from build123d import *

# Parameters (mm, degrees)
SKETCH1_W           = 180
SKETCH1_H           = 70
BOSS_EXTRUDE1_DEPTH = 3
SKETCH2_W           = 3
SKETCH2_H           = 27
SKETCH2_W_2         = 40
SKETCH2_H_2         = 3
CUT_EXTRUDE6_DEPTH  = 10
SKETCH3_R           = 5
CUT_EXTRUDE7_DEPTH  = 12


with BuildPart() as part:
    # Sketch1 → Boss-Extrude1 (new body)
    with BuildSketch(Plane(origin=(0, 0, 0), x_dir=(0, 0, -1), z_dir=(1, 0, 0))):
        Rectangle(SKETCH1_W, SKETCH1_H)
    extrude(amount=BOSS_EXTRUDE1_DEPTH)

    # Sketch2 → Cut-Extrude6 (cut)
    with BuildSketch(Plane(origin=(3, 0, 0), x_dir=(0, 0, -1), z_dir=(1, 0, 0))):
        Polygon((90, -32), (87, -32), (55, -32), (55, -35), (90, -35), align=None)
        with Locations((88.5, -18.5)):
            Rectangle(SKETCH2_W, SKETCH2_H)
        with Locations((25, -33.5)):
            Rectangle(SKETCH2_W_2, SKETCH2_H_2)
        with Locations((-25, -33.5)):
            Rectangle(SKETCH2_W_2, SKETCH2_H_2)
        Polygon((-55, -32), (-87, -32), (-90, -32), (-90, -35), (-55, -35), align=None)
        with Locations((-88.5, -18.5)):
            Rectangle(SKETCH2_W, SKETCH2_H)
        with Locations((-88.5, 18.5)):
            Rectangle(SKETCH2_W, SKETCH2_H)
        Polygon((-87, 32), (-55, 32), (-55, 35), (-90, 35), (-90, 32), align=None)
        with Locations((-25, 33.5)):
            Rectangle(SKETCH2_W_2, SKETCH2_H_2)
        with Locations((25, 33.5)):
            Rectangle(SKETCH2_W_2, SKETCH2_H_2)
        Polygon((55, 32), (87, 32), (90, 32), (90, 35), (55, 35), align=None)
        with Locations((88.5, 18.5)):
            Rectangle(SKETCH2_W, SKETCH2_H)
    extrude(amount=-CUT_EXTRUDE6_DEPTH, mode=Mode.SUBTRACT)

    # Sketch3 → Cut-Extrude7 (cut)
    with BuildSketch(Plane(origin=(3, 0, 0), x_dir=(0, 0, -1), z_dir=(1, 0, 0))):
        with Locations((-69.072414396, 17.873185396)):
            Circle(SKETCH3_R)
    extrude(amount=-CUT_EXTRUDE7_DEPTH, mode=Mode.SUBTRACT)


solid = part.part
Read the model definition and answer for the solid it produces. Units are mm, in the model's axes. A direction names the side the tool comes from. Give positions to 0.01 mm unless a question says otherwise; leave off trailing zeros. Write each loop counter-clockwise with the first axis right and the second up, starting at its lowest first coordinate (ties: lowest second). Pieces come first, ordered by that corner, then holes. Notation, with made-up numbers: (89.25, 68) - (129.25, 68) arc R23 ccw to (129.25, 94) - close; hole circle Ø10 at (53.25, 61.25). An arc over 180 degrees is marked (long way). Use CSV: the item, a comma, the result in double quotes. Start each with the question number.
(1) Consider line 1 along Z through (x, y) = (2.05, 18); line 2 along Z through (x, y) = (2.4, 30.5); line 3 along Y through (x, z) = (2.15, -10). Determine where each line is inside the solid, lowest interval first.
(2) For faces 1 (the flat face through (2, -34, -45)), 2 (the flat face through (2, 32, -71)), 3 (the flat face through (2, -19, -87)), 4 (the flat face through (2, 33, -5)), determine the directions among +Z, -Z, +X, -X, +Y, -Y from which every point of the face is accessible in a straight line to the end or side of a thin tool.
(3) Find section A-A (y = 15). Give the vertices of the cut face in (x, z), plus the area to 3 significant figures.
(4) Given P1, Ø1, axis at x = 0.5, y = 7.5, coming from the -Z side; P2, Ø1, axis at x = 1, z = 68, coming from the +Y side; P3, Ø0.9, axis at x = 1.5, z = 88, coming from the -Y side, each flat-ended and moving along its own axis, determine where each tip first touches the part or whether it passes through.
(5) Find section B-B (z = -10). Give the vertices of the cut face in (x, y).
(6) Determine the mould class of faces 5 (the flat face through (2, -34, 5)), 6 (the flat face through (2, -19, 87)), 7 (the flat face through (2, 18, -87)) for opening direction Z: +Z half, -Z half, draft (parallel to the pull), parting line (faces both ways), or undercut.
Findings below:
1,line 1,"-87 to 64.07, 74.07 to 87"
1,line 2,"-87 to 87"
1,line 3,"-32 to 32"
2,face 1,"+X, -X, -Y"
2,face 2,"-Z, +X, -X, +Y"
2,face 3,"-Z, +X, -X, -Y"
2,face 4,"+X, -X, +Y"
3,outline,"(0, -87) - (3, -87) - (3, 64.98) - (0, 64.98) - close; (0, 73.16) - (3, 73.16) - (3, 87) - (0, 87) - close"
3,area,"497 mm2"
4,P1,"z = -87"
4,P2,"y = 32"
4,P3,"y = -5"
5,outline,"(0, -32) - (3, -32) - (3, 32) - (0, 32) - close"
6,face 5,"undercut"
6,face 6,"+Z half"
6,face 7,"-Z half"
